Part model, mm, in its own coordinate system. A direction names the side the tool comes from. Give positions to 0.01 mm unless a question says otherwise; leave off trailing zeros. Write each loop counter-clockwise with the first axis right and the second up, starting at its lowest first coordinate (ties: lowest second). Pieces come first, ordered by that corner, then holes.
Autodesk Fusion 360 part; units mm, degrees
sketch "Sketch1" plane through (0, 0, 0) normal (0, 1, 0) x (1, 0, 0)
  line L0 (3.75, -72) -> (-3.75, -72)
  line L1 (-3.75, -72) -> (-3.75, 72)
  line L2 (-3.75, 72) -> (3.75, 72)
  line L3 (3.75, 72) -> (3.75, -72)
  line L4 (3.75, -72) -> (-3.75, 72) construction
  line L5 (-3.75, -72) -> (3.75, 72) construction
  dimension "d1" = 7.5
  dimension "d2" = 144
extrude "Extrude1" add sketch "Sketch1" along normal blind 5
sketch "Sketch2" plane through (0, 5, 0) normal (0, 1, 0) x (-1, 0, 0)
  line L0 (-3.75, -72) -> (3.75, -72)
  line L1 (3.75, -72) -> (3.75, 72)
  line L2 (3.75, 72) -> (-3.75, 72)
  line L3 (-3.75, 72) -> (-3.75, -72)
  line L4 (3.75, 72) -> (-3.75, 72)
  line L5 (-3.75, 72) -> (-3.75, 67)
  line L6 (-3.75, 67) -> (3.75, 67)
  line L7 (3.75, 67) -> (3.75, 72)
  dimension "d5" = 5
extrude "Extrude2" add sketch "Sketch2" along normal blind 10 contours L1 L2 L3 L4 L5 L6 L7
sketch "Sketch3" plane through (0, 5, 0) normal (0, 1, 0) x (-1, 0, 0)
  line L0 (3.75, 67) -> (-3.75, 67)
  line L1 (-3.75, 67) -> (-3.75, -72)
  line L2 (-3.75, -72) -> (3.75, -72)
  line L3 (3.75, -72) -> (3.75, 67)
  line L4 (3.75, -72) -> (-3.75, -72)
  line L5 (-3.75, -72) -> (-3.75, -67)
  line L6 (-3.75, -67) -> (3.75, -67)
  line L7 (3.75, -67) -> (3.75, -72)
  dimension "d8" = 5
extrude "Extrude3" add sketch "Sketch3" along normal blind 10 contours L1 L2 L3 L4 L5 L6 L7
fillet "Fillet1" radius 5 1 edges at (0, 15, 72)
fillet "Fillet2" radius 5 1 edges at (0, 15, -72)
sketch "Sketch6" plane through (0, 5, 0) normal (0, 1, 0) x (-1, 0, 0)
  line L0 (-3.75, -67) -> (3.75, -67)
  line L1 (3.75, -67) -> (3.75, 67)
  line L2 (3.75, 67) -> (-3.75, 67)
  line L3 (-3.75, 67) -> (-3.75, -67)
  line L4 (3.75, -67) -> (1, -67)
  line L5 (1, -67) -> (1, -64.5)
  line L6 (1, -64.5) -> (3.75, -64.5)
  line L7 (3.75, -64.5) -> (3.75, -67)
  line L8 (-3.75, -67) -> (-1, -67)
  line L9 (-1, -67) -> (-1, -64.5)
  line L10 (-1, -64.5) -> (-3.75, -64.5)
  line L11 (-3.75, -64.5) -> (-3.75, -67)
  dimension "d18" = 2.75
  dimension "d19" = 2.5
  dimension "d20" = 2.75
  dimension "d21" = 2.5
extrude "Extrude5" add sketch "Sketch6" along normal blind 10 contours L0 L3 L8 L9 L10 L11 | L0 L1 L4 L5 L6 L7
sketch "Sketch7" plane through (0, 5, 0) normal (0, 1, 0) x (-1, 0, 0)
  line L0 (1, -67) -> (1, -64.5)
  line L1 (1, -64.5) -> (3.75, -64.5)
  line L2 (3.75, -64.5) -> (3.75, 67)
  line L3 (3.75, 67) -> (-3.75, 67)
  line L4 (-3.75, 67) -> (-3.75, -64.5)
  line L5 (-3.75, -64.5) -> (-1, -64.5)
  line L6 (-1, -64.5) -> (-1, -67)
  line L7 (-1, -67) -> (1, -67)
  line L8 (-3.75, 67) -> (-1, 67)
  line L9 (-1, 67) -> (-1, 64.5)
  line L10 (-1, 64.5) -> (-3.75, 64.5)
  line L11 (-3.75, 64.5) -> (-3.75, 67)
  dimension "d24" = 2.75
  dimension "d25" = 2.5
sketch "Sketch8" plane through (0, 5, 0) normal (0, 1, 0) x (-1, 0, 0)
  line L0 (3.75, 67) -> (1, 67)
  line L1 (1, 67) -> (1, 64.5)
  line L2 (1, 64.5) -> (3.75, 64.5)
  line L3 (3.75, 64.5) -> (3.75, 67)
  point P0 (3.75, 67)
  dimension "d26" = 2.75
  dimension "d27" = 2.5
extrude "Extrude6" add sketch "Sketch8" sketch "Sketch7" along normal blind 10 of sketch 2 contours L3 L4 L8 L9 L10 L11
sketch "Sketch9" plane through (0, 5, 0) normal (0, 1, 0) x (-1, 0, 0)
  line L0 (-1, 67) -> (-1, 64.5)
  line L1 (-1, 64.5) -> (-3.75, 64.5)
  line L2 (-3.75, 64.5) -> (-3.75, -64.5)
  line L3 (-3.75, -64.5) -> (-1, -64.5)
  line L4 (-1, -64.5) -> (-1, -67)
  line L5 (-1, -67) -> (1, -67)
  line L6 (1, -67) -> (1, -64.5)
  line L7 (1, -64.5) -> (3.75, -64.5)
  line L8 (3.75, -64.5) -> (3.75, 64.5)
  line L9 (3.75, 64.5) -> (1, 64.5)
  line L10 (1, 64.5) -> (1, 67)
  line L11 (1, 67) -> (-1, 67)
  line L12 (-3.75, 64.5) -> (-1, 64.5)
  line L13 (-1, 64.5) -> (-1, 14.5)
  line L14 (-1, 14.5) -> (-3.75, 14.5)
  line L15 (-3.75, 14.5) -> (-3.75, 64.5)
  line L16 (3.75, 64.5) -> (1, 64.5)
  line L17 (1, 64.5) -> (1, 14.5)
  line L18 (1, 14.5) -> (3.75, 14.5)
  line L19 (3.75, 14.5) -> (3.75, 64.5)
  line L20 (3.75, -64.5) -> (1, -64.5)
  line L21 (1, -64.5) -> (1, -14.5)
  line L22 (1, -14.5) -> (3.75, -14.5)
  line L23 (3.75, -14.5) -> (3.75, -64.5)
  line L24 (-3.75, -64.5) -> (-1, -64.5)
  line L25 (-1, -64.5) -> (-1, -14.5)
  line L26 (-1, -14.5) -> (-3.75, -14.5)
  line L27 (-3.75, -14.5) -> (-3.75, -64.5)
  dimension "d30" = 2.75
  dimension "d31" = 50
  dimension "d32" = 2.75
  dimension "d33" = 50
  dimension "d34" = 2.75
  dimension "d35" = 50
  dimension "d36" = 2.75
  dimension "d37" = 50
extrude "Extrude7" add sketch "Sketch9" along normal blind 3 contours L1 L2 L12 L13 L14 L15 | L8 L9 L16 L17 L18 L19 | L2 L3 L24 L25 L26 L27 | L7 L8 L20 L21 L22 L23
fillet "Fillet3" radius 3 4 edges at (2.375, 8, -14.5) (-2.375, 8, -14.5) (-2.375, 8, 14.5) (2.375, 8, 14.5)
fillet "Fillet4" radius 1 4 edges at (-2.375, 15, 64.5) (2.375, 15, 64.5) (-2.375, 15, -64.5) (2.375, 15, -64.5)
fillet "Fillet5" radius 1 4 edges at (-2.375, 8, -64.5) (2.375, 8, -64.5) (2.375, 8, 64.5) (-2.375, 8, 64.5)
fillet "Fillet6" radius 2 1 edges at (0, 0, -72)
fillet "Fillet7" radius 2 1 edges at (0, 0, 72)
fillet "Fillet8" radius 0.5 20 edges at (-3.75, 7.1213, 15.3787) (-3.75, 8, 40.5) (-3.75, 8.2929, 64.2071) (-3.75, 11.5, 64.5) (-3.75, 14.7071, 64.7929) (-3.75, 15, 66.25) (-3.75, 13.5355, 70.5355) (-3.75, 6, 72) (-3.75, 0.5858, 71.4142) (-3.75, 0, 0) (-3.75, 0.5858, -71.4142) (-3.75, 6, -72) (-3.75, 13.5355, -70.5355) (-3.75, 15, -66.25) (-3.75, 14.7071, -64.7929) (-3.75, 11.5, -64.5) (-3.75, 8.2929, -64.2071) (-3.75, 8, -40.5) (-3.75, 7.1213, -15.3787) (-3.75, 5, 0)
fillet "Fillet9" radius 0.5 20 edges at (3.75, 7.1213, -15.3787) (3.75, 8, -40.5) (3.75, 8.2929, -64.2071) (3.75, 11.5, -64.5) (3.75, 14.7071, -64.7929) (3.75, 15, -66.25) (3.75, 13.5355, -70.5355) (3.75, 6, -72) (3.75, 0.5858, -71.4142) (3.75, 0, 0) (3.75, 0.5858, 71.4142) (3.75, 6, 72) (3.75, 13.5355, 70.5355) (3.75, 15, 66.25) (3.75, 14.7071, 64.7929) (3.75, 11.5, 64.5) (3.75, 8.2929, 64.2071) (3.75, 8, 40.5) (3.75, 7.1213, 15.3787) (3.75, 5, 0)
1) Flat gauge pins, fed straight in: P1, Ø1, axis at x = 0, y = 11, coming from the +Z side; P2, Ø0.7, axis at x = 2.5, z = 35.5, coming from the +Y side; P3, Ø1.8, axis at x = 1.5, y = 12, coming from the -Z side. Where does each tip first touch, or does it go through?
Check result:
P1: stops at z = 71.98
P2: stops at y = 8
P3: stops at z = -71.88
2) Saw through at A-A (z = -29). Write the cut outline in (x, y), and give its area (3 significant figures).
Check result:
outline: (-3.75, 0.5) arc R0.5 ccw to (-3.25, 0) - (3.25, 0) arc R0.5 ccw to (3.75, 0.5) - (3.75, 7.5) arc R0.5 ccw to (3.25, 8) - (1, 8) - (1, 5) - (-1, 5) - (-1, 8) - (-3.25, 8) arc R0.5 ccw to (-3.75, 7.5) - close
area: 53.8 mm2
3) Drill centre lines: L1, parallel to Z at x = 3.25, y = 14; L2, parallel to Z at x = -2.5, y = 9.25; L3, parallel to Y at x = -0.5, z = -44.5. Where is each one in solid material? Low to high.
Check result:
L1: z = -70 to -64.5, 64.5 to 70
L2: z = -72 to -64.5, 64.5 to 72
L3: y = 0 to 5
4) 3-axis set-ups, long thin cutter, end or side, ignore diameter. For faces 1 (the cylindrical face through (2.14, 7.1, 15.36)), 2 (the flat face through (-3.75, 4, -1)), 3 (the flat face through (-1, 7, 43)): which of +Z, -Z, +X, -X, +Y, -Y reach the whole face in a straight line?
Check result:
face 1: +X, -X, +Y
face 2: +Z, -Z, -X, +Y, -Y
face 3: +Y
5) Saw through at B-B (z = -10). Write the cut outline in (x, y).
Check result:
outline: (-3.75, 0.5) arc R0.5 ccw to (-3.25, 0) - (3.25, 0) arc R0.5 ccw to (3.75, 0.5) - (3.75, 4.5) arc R0.5 ccw to (3.25, 5) - (-3.25, 5) arc R0.5 ccw to (-3.75, 4.5) - close
